Source: CAD feature listing. Evaluate the final solid. Frame: model axes, mm. A direction names the side the tool comes from. Coordinates: 2 decimals unless noted, no trailing zeros. Write item = value, one per line. Start each with the question number.
from build123d import *

# Parameters (mm, degrees)
SKETCH2_W           = 33
SKETCH2_H           = 28
BOSS_EXTRUDE1_DEPTH = 46
SKETCH3_W           = 17.5
SKETCH3_H           = 41
CUT_EXTRUDE1_DEPTH  = 46
BOSS_EXTRUDE2_DEPTH = 3
BOSS_EXTRUDE3_REACH = 58.675
FILLET1_START       = -3.5
FILLET1_DEPTH       = 4.934820146
FILLET1_START_2     = -13.5
FILLET1_2_DEPTH     = 27
FILLET2_R           = 16.5
FILLET3_R           = 6
SKETCH6_W           = 13
SKETCH6_H           = 23
CUT_EXTRUDE2_DEPTH  = 9
SKETCH7_R           = 6.5
CUT_EXTRUDE3_DEPTH  = 9
SKETCH8_R           = 1
CUT_EXTRUDE4_DEPTH  = 8
SKETCH9_R           = 1.3
SKETCH9_R_2         = 2.5
CUT_EXTRUDE5_DEPTH  = 47.360004726


with BuildPart() as part:
    # Sketch2 → Boss-Extrude1 (new body)
    with BuildSketch(Plane(origin=(0, 0, 0), x_dir=(1, 0, 0), z_dir=(0, 1, 0))):
        Rectangle(SKETCH2_W, SKETCH2_H)
    extrude(amount=BOSS_EXTRUDE1_DEPTH)

    # Sketch3 → Cut-Extrude1 (cut)
    with BuildSketch(Plane(origin=(16.5, 0, 0), x_dir=(0, 0, -1), z_dir=(1, 0, 0))):
        with Locations((-5.25, 25.5)):
            Rectangle(SKETCH3_W, SKETCH3_H)
    extrude(amount=-CUT_EXTRUDE1_DEPTH, mode=Mode.SUBTRACT)

    # Sketch4 → Boss-Extrude2 (add)
    with BuildSketch(Plane(origin=(16.5, 0, 0), x_dir=(0, 0, -1), z_dir=(1, 0, 0))):
        with BuildLine():
            Line((3.5, 46), (2, 46))
            add(Edge.make_bspline(
                [(-14, 5), (-0.513369381, 23.145305793), (2, 46)],
                knots=[0, 0, 0, 1, 1, 1], degree=2))
            Line((-14, 5), (3.5, 5))
            Line((3.5, 5), (3.5, 46))
        make_face()
    boss_extrude2 = extrude(amount=-BOSS_EXTRUDE2_DEPTH)

    # Mirror1: Boss-Extrude2 across plane
    add(boss_extrude2.mirror(Plane(origin=(0, 0, 0), x_dir=(0, 0, 1), z_dir=(1, 0, 0))))

    # Boss-Extrude3: up to this face of the body (flat: up to its plane)
    boss_extrude3_end = Plane(part.part.faces().sort_by_distance((-13.5, 18.213858907, 1.639358486))[0])
    # Sketch5 → Boss-Extrude3 (add, up to the picked face)
    with BuildSketch(Plane.ZY.offset(-13.5), mode=Mode.PRIVATE) as boss_extrude3_sk1:
        with BuildLine():
            Line((-3.5, 43), (-1.619905063, 43))
            add(Edge.make_bspline(
                [(-1.619905063, 43), (-1.833911679, 44.489717492), (-2.000000005, 46.00000005)],
                knots=[0, 0, 0, 1, 1, 1], degree=2))
            Line((-2.000000005, 46.00000005), (-3.5, 46))
            Line((-3.5, 46), (-3.5, 43))
        make_face()
    boss_extrude3_tool1 = split(extrude(boss_extrude3_sk1.sketch, amount=BOSS_EXTRUDE3_REACH, mode=Mode.PRIVATE), bisect_by=boss_extrude3_end, keep=Keep.BOTH, mode=Mode.PRIVATE)
    add(boss_extrude3_tool1.solids().sort_by(Axis((13.5, 44.443503, -2.655604), (-1, 0, 0)))[0])

    # Fillet1: read off the stored shape, not the designer's step
    # Fillet1 outline → Fillet1 (add)
    with BuildSketch(Plane.XY.offset(FILLET1_START)):
        with BuildLine():
            ThreePointArc((-13.5, 29.5), (-9.545941546, 39.045941546), (0, 43))
            Line((0, 43), (-13.5, 43))
            Line((-13.5, 43), (-13.5, 29.5))
        make_face()
        with BuildLine():
            ThreePointArc((0, 43), (9.545941546, 39.045941546), (13.5, 29.5))
            Line((13.5, 29.5), (13.5, 43))
            Line((13.5, 43), (0, 43))
        make_face()
    extrude(amount=FILLET1_DEPTH)

    # Fillet1 2 outline → Fillet1 2 (cut)
    with BuildSketch(Plane.YZ.offset(FILLET1_START_2)):
        with BuildLine():
            Line((43, 1.434820146), (29.5, 1.434820046))
            add(Edge.make_bspline(
                [(29.5, 1.434820046), (36.024557501, -0.617842021), (43, -1.619905063)],
                knots=[0.500321207, 0.500321207, 0.500321207, 0.500855825, 0.500855825, 0.500855825], degree=2))
            Line((43, -1.619905063), (43, 1.434820146))
        make_face()
    extrude(amount=FILLET1_2_DEPTH, mode=Mode.SUBTRACT)

    # Fillet2
    # the kernel refuses this fillet: 16.5 mm, written as the material it takes off along each edge
    with BuildSketch(Plane(origin=(16.5, 46, -55.25), x_dir=(0, -1, 0), z_dir=(0, 0, 1)), Plane(origin=(-16.5, 46, 39.25), x_dir=(0, -1, 0), z_dir=(0, 0, -1))) as fillet2_piece_1:
        with BuildLine():
            CenterArc((FILLET2_R, -FILLET2_R), FILLET2_R, 90, 90)
            Line((0, -FILLET2_R), (0, 0))
            Line((0, 0), (FILLET2_R, 0))
        make_face()
    extrude(amount=94.5, mode=Mode.SUBTRACT)

    # Fillet3
    # the kernel refuses this fillet: 6 mm, written as the material it takes off along each edge
    with BuildSketch(Plane(origin=(-16.5, -15, 14), x_dir=(1, 0, 0), z_dir=(0, 1, 0)), Plane(origin=(16.5, -15, 14), x_dir=(0, 0, -1), z_dir=(0, 1, 0))) as fillet3_piece_1:
        with BuildLine():
            CenterArc((FILLET3_R, FILLET3_R), FILLET3_R, 180, 90)
            Line((0, FILLET3_R), (0, 0))
            Line((0, 0), (FILLET3_R, 0))
        make_face()
    extrude(amount=35, mode=Mode.SUBTRACT)

    # Sketch6 → Cut-Extrude2 (cut)
    with BuildSketch(Plane.XY.offset(-3.5)):
        with Locations((0, 23)):
            Rectangle(SKETCH6_W, SKETCH6_H)
    extrude(amount=-CUT_EXTRUDE2_DEPTH, mode=Mode.SUBTRACT)

    # Sketch7 → Cut-Extrude3 (cut)
    with BuildSketch(Plane.XY.offset(-12.5)):
        with Locations((0, 28)):
            Circle(SKETCH7_R)
    extrude(amount=-CUT_EXTRUDE3_DEPTH, mode=Mode.SUBTRACT)

    # Sketch8 → Cut-Extrude4 (cut)
    with BuildSketch(Plane.XY.offset(-3.5)):
        with Locations((0, 36.8)):
            Circle(SKETCH8_R)
        with Locations((0, 9.2)):
            Circle(SKETCH8_R)
    extrude(amount=-CUT_EXTRUDE4_DEPTH, mode=Mode.SUBTRACT)

    # Sketch9 → Cut-Extrude5 (cut, through all)
    with BuildSketch(Plane(origin=(0, 5, 0), x_dir=(1, 0, 0), z_dir=(0, 1, 0))):
        with Locations(Location((-0.5, 0, 0), (0, 0, 270))):
            Circle(SKETCH9_R)
        with Locations(Location((-5, 0, 0), (0, 0, 270))):
            Circle(SKETCH9_R_2)
        with Locations(Location((-9.5, 0, 0), (0, 0, 270))):
            Circle(SKETCH9_R)
    extrude(amount=-CUT_EXTRUDE5_DEPTH, mode=Mode.SUBTRACT)


solid = part.part
Item 1: Reachability of faces 1 (the flat face through (6.5, 23, -8)), 2 (the flat face through (-16.5, 15, -3)) from +Z, -Z, +X, -X, +Y, -Y: full face, straight path, thin tool, end or side. Return the list, or none.
Item 2: Material intervals for L1, parallel to X at y = 3.1, z = 0; L2, parallel to Y at x = 0, z = -7.5; L3, parallel to Y at x = 0, z = -13, sorted ascending. Write a range as [from, to].
Item 3: Draft query along Y for faces 3 (the flat face through (-13.5, 15, 3)), 4 (the flat face through (0, 18, -14)), 5 (the flat face through (0, 0, -3)). Return one class per face: released by +Y, released by -Y, zero draft, split by the parting line, or undercut.
Item 4: First-contact query: pin 1 (14.5 mm diameter, centred on x = -2.5, y = 18, fed in from +Z); pin 2 (1.5 mm diameter, centred on x = -4, y = 17.5, fed in from +Z); pin 3 (5 mm diameter, centred on x = 3, z = 3.5, fed in from +Y); pin 4 (1.6 mm diameter, centred on x = -0.5, z = 0, fed in from +Y). Flat tips, straight axial feed; report the tip coordinate or a pass-through.
Responses:
q1.face_1 = +Z
q1.face_2 = +Z, -Z, -X, +Y, -Y
q2.L1 = [-16.5, -10.8], [-8.2, -7.5], [-2.5, -1.8], [0.8, 16.5]
q2.L2 = [0, 8.2], [10.2, 11.5], [34.5, 35.8], [37.8, 46]
q2.L3 = [0, 21.5], [34.5, 46]
q3.face_3 = undercut
q3.face_4 = zero draft
q3.face_5 = released by -Y
q4.pin_1 = -3.5
q4.pin_2 = -12.5
q4.pin_3 = 5
q4.pin_4 = through
